from build123d import *

# Parameters (mm, degrees)
CUT_EXTRUDE1_DEPTH = 9.525
CHAMFER1_SIZE      = 0.9525


with BuildPart() as part:
    # Sketch1 → Revolve1 (revolve)
    with BuildSketch(Plane.XY, mode=Mode.PRIVATE) as revolve1_sk:
        Polygon((0, 0), (100.6348, 0), (100.6348, 5.969), (79.5528, 5.969), (79.5528, 10.033), (7.9248, 10.033), (7.9248, 6.858), (4.7498, 6.858), (4.7498, 10.033), (0, 10.033), align=None)
    revolve(revolve1_sk.sketch.rotate(Axis((0, 0, 0), (1, 0, 0)), 180), axis=Axis((0, 0, 0), (1, 0, 0)))

    # Sketch2 → Cut-Extrude1 (cut)
    with BuildSketch(Plane(origin=(100.6348, 0, 0), x_dir=(0, 0, -1), z_dir=(1, 0, 0))):
        Polygon((3.666174209, 0), (1.833087105, 3.175), (-1.833087105, 3.175), (-3.666174209, 0), (-1.833087105, -3.175), (1.833087105, -3.175), align=None)
    extrude(amount=-CUT_EXTRUDE1_DEPTH, mode=Mode.SUBTRACT)

    # Chamfer1
    chamfer1_edges = [part.edges().sort_by_distance(p)[0] for p in [
        (100.6348, 5.969, 0),
        (0, 10.033, 0),
    ]]
    chamfer(chamfer1_edges, length=CHAMFER1_SIZE)


solid = part.part
Part model, mm, in its own coordinate system. A direction names the side the tool comes from. Round coordinates to 2 decimals unless told otherwise and drop trailing zeros. Write each loop counter-clockwise with the first axis right and the second up, starting at its lowest first coordinate (ties: lowest second). Pieces come first, ordered by that corner, then holes. Notation, with made-up numbers: (70, 38) - (116, 38) arc R19 ccw to (116, 47) - close; hole circle Ø1 at (80, -2.5). An arc over 180 degrees is marked (long way). Use CSV: the item, a comma, the result in double quotes.
Item 1: Slice it at A-A, the plane x = 36.5. Write the cut outline in (y, z), then the cut area to 3 significant figures.
Results list:
outline,"circle Ø20.07 at (0, 0)"
area,"316 mm²"
Item 2: Flat gauge pins, fed straight in: P1, Ø10, axis at x = 26.5, z = 6, coming from the -Y side; P2, Ø1.5, axis at x = 60.5, z = 5.5, coming from the -Y side; P3, Ø5, axis at x = 52.5, y = -3.5, coming from the -Z side. Where does each tip first touch, or does it go through?
Results list:
P1,"stops at y = -9.98"
P2,"stops at y = -8.84"
P3,"stops at z = -9.98"
Item 3: Wall check: L1, parallel to X at y = 3, z = -7; L2, parallel to Z at x = 92, y = 1.5; L3, parallel to X at y = 6, z = 1.5. Give the ranges that are in metal, low to high.
Results list:
L1,"x = 0 to 4.75, 7.92 to 79.55"
L2,"z = -5.78 to -2.8, 2.8 to 5.78"
L3,"x = 0 to 79.55"
Item 4: Tool access for faces 5 (the cylindrical face through (43.237, 2.175, 9.794)), 6 (the flat face through (96, -3.175, 0)), 7 (the flat face through (7.925, -2, 7)): list every direction of +Z, -Z, +X, -X, +Y, -Y with a clear straight run to the whole face (end or side of a thin tool).
Results list:
face 5,"+X, -X"
face 6,"+X"
face 7,"none"
Item 5: Pull direction Z, two halves, no side cores. Call faces 1 (the flat face through (95.94, -1.57, 2.76)), 2 (the flat face through (91.11, 0, 0)), 3 (the cylindrical face through (6.315, 1.487, 6.695)), 4 (the flat face through (100.635, 1, 3.3)): pulls with the +Z half, pulls with the -Z half, needs draft (parallel to the pull), parting line crosses it, or undercut.
Results list:
face 1,"undercut"
face 2,"undercut"
face 3,"parting line crosses it"
face 4,"needs draft"
